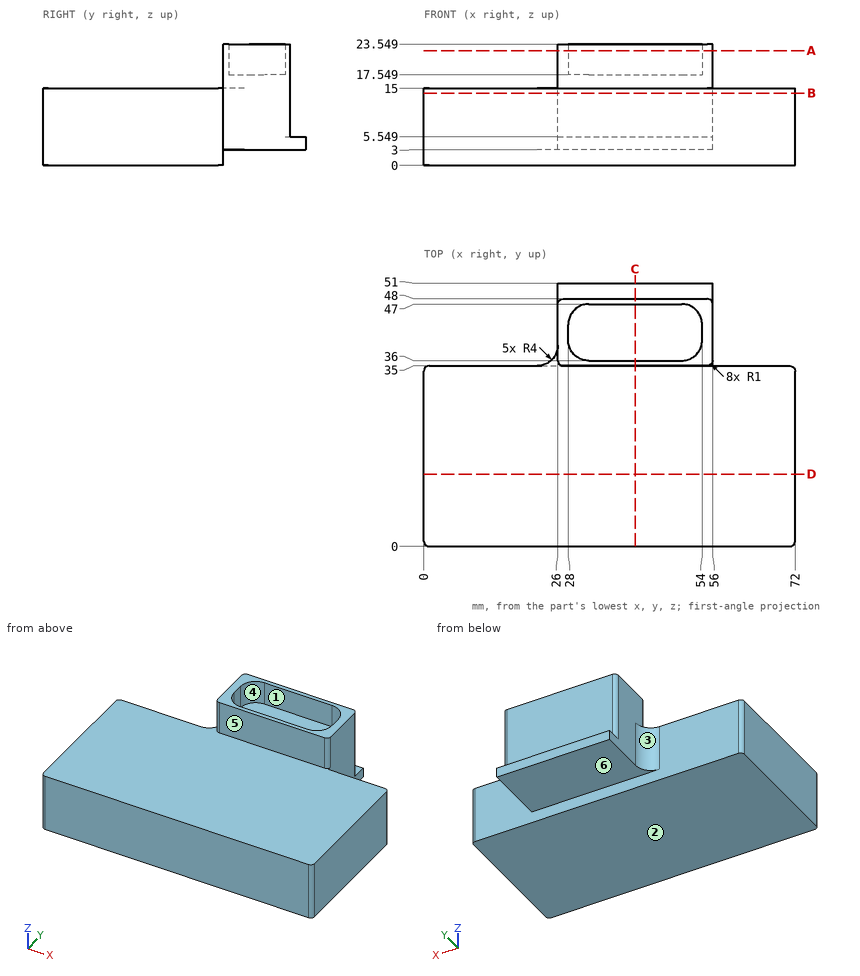
Part print with two shaded views. Sizes in mm from the minimum x, y, z corner. A direction names the side the tool comes from. Round coordinates to 2 decimals unless told otherwise and drop trailing zeros. Order: outer loops, then holes, each group sorted by start corner. A loop starts at its lowest first (then second) coordinate and runs counter-clockwise, first axis right, second up.
(1) Band-saw the part on B-B (z = 14). List the corners of the cut face in (x, y), then the cut area to 3 significant figures.
(2) Band-saw the part on C-C (x = 41). List the corners of the cut face in (y, z), then the cut area to 3 significant figures.
(3) Pin check, flat tips, straight feed: pin 1 (0.9 mm diameter, centred on y = 41.5, z = 21, fed in from -X); pin 2 (9.5 mm diameter, centred on x = 46.5, z = 20, fed in from -Y); pin 3 (3.5 mm diameter, centred on x = 45.5, y = 39.5, fed in from +Z). Stop position of each tip, or through.
(4) Band-saw the part on D-D (y = 14). List the corners of the cut face in (x, z).
(5) Band-saw the part on A-A (z = 22.25). List the corners of the cut face in (x, y), then the cut area to 3 significant figures.
(6) Drill centre lines: line 1 (Y direction, x = 48.5, z = 7.25); line 2 (Z direction, x = 14, y = 26.5); line 3 (Y direction, x = 47.5, z = 17.75). Where is each one in solid material? Low to high.
(7) 3-axis set-ups, long thin cutter, end or side, ignore diameter. For the marked faces 4, 5 and 6: which of +Z, -Z, +X, -X, +Y, -Y reach the whole face in a straight line?
(8) Pull direction Y, two halves, no side cores. Call the marked faces 1, 2 and 3: released by +Y, released by -Y, zero draft, split by the parting line, or undercut.
Verdict:
1. outline: (0, 1) arc R1 ccw to (1, 0) - (71, 0) arc R1 ccw to (72, 1) - (72, 34) arc R1 ccw to (71, 35) - (56, 35) - (56, 47) arc R1 ccw to (55, 48) - (27, 48) arc R1 ccw to (26, 47) - (26, 39) arc R4 cw to (22, 35) - (1, 35) arc R1 ccw to (0, 34) - close
1. area: 2,910 mm2
2. outline: (0, 0) - (35, 0) - (35, 3) - (51, 3) - (51, 5.55) - (48, 5.55) - (48, 23.55) - (47, 23.55) - (47, 17.55) - (36, 17.55) - (36, 23.55) - (35, 23.55) - (35, 15) - (0, 15) - close
2. area: 734 mm2
3. pin 1: stops at x = 26
3. pin 2: stops at y = 35
3. pin 3: stops at z = 17.55
4. outline: (0, 0) - (72, 0) - (72, 15) - (0, 15) - close
5. outline: (26, 36) arc R1 ccw to (27, 35) - (55, 35) arc R1 ccw to (56, 36) - (56, 47) arc R1 ccw to (55, 48) - (27, 48) arc R1 ccw to (26, 47) - close; hole (28, 40) arc R4 ccw to (32, 36) - (50, 36) arc R4 ccw to (54, 40) - (54, 43) arc R4 ccw to (50, 47) - (32, 47) arc R4 ccw to (28, 43) - close
5. area: 117 mm2
6. line 1: y = 0 to 48
6. line 2: z = 0 to 15
6. line 3: y = 35 to 36, 47 to 48
7. face 4: +Z
7. face 5: +Z, +X, -X, -Y
7. face 6: -Z, +X, -X, +Y
8. face 1: undercut
8. face 2: zero draft
8. face 3: released by +Y
